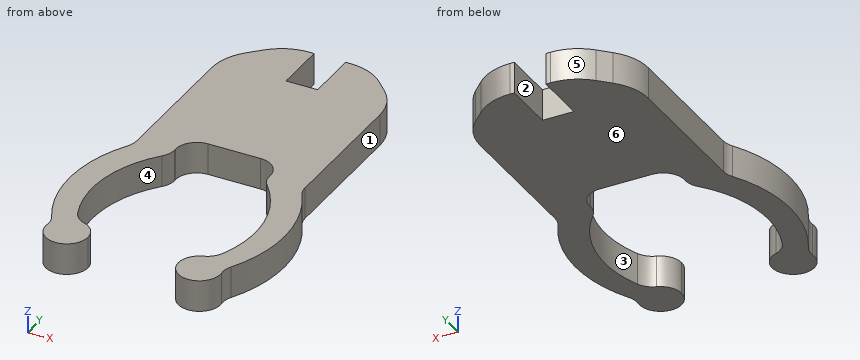
from build123d import *

# Parameters (mm, degrees)
F2_DEPTH = 1.5
F5_W     = 3
F5_H     = 5
F6_DEPTH = 25
F7_SIZE  = 4
F8_R     = 5
F9_R     = 2


with BuildPart() as f2:
    # F1 (on Top) → F2 (new body, symmetric)
    with BuildSketch(Plane.XY):
        with BuildLine():
            ThreePointArc((25.939839122, -44.6497348995), (25.3779596461, -43.9442064652), (24.8663520645, -43.2014167241))
            ThreePointArc((24.8663520645, -43.2014167241), (26.2921371989, -45.9579703612), (28.7, -44))
            ThreePointArc((28.7, -44), (28.0793670217, -42.5517781181), (26.6026533807, -42.0023704959))
            ThreePointArc((26.6026533807, -42.0023704959), (27.0242100762, -42.7170517529), (27.4984385882, -43.3979237417))
            ThreePointArc((27.4984385882, -43.3979237417), (27.6482717407, -43.6825402295), (27.7, -44))
            ThreePointArc((27.7, -44), (27.0462940384, -44.9381260251), (25.939839122, -44.6497348995))
        make_face()
        with BuildLine():
            ThreePointArc((27.4984385882, -43.3979237417), (26.0738018768, -43.2203360272), (25.939839122, -44.6497348995))
            ThreePointArc((25.939839122, -44.6497348995), (27.0462940384, -44.9381260251), (27.7, -44))
            ThreePointArc((27.7, -44), (27.6482717407, -43.6825402295), (27.4984385882, -43.3979237417))
        make_face()
        with BuildLine():
            ThreePointArc((26.6026533807, -42.0023704959), (25.5635084879, -42.3542822104), (24.8663520645, -43.2014167241))
            ThreePointArc((24.8663520645, -43.2014167241), (25.3779596461, -43.9442064652), (25.939839122, -44.6497348995))
            ThreePointArc((25.939839122, -44.6497348995), (26.0738018768, -43.2203360272), (27.4984385882, -43.3979237417))
            ThreePointArc((27.4984385882, -43.3979237417), (27.0242100762, -42.7170517529), (26.6026533807, -42.0023704959))
        make_face()
        with BuildLine():
            Line((28.5, -29), (25, -29))
            ThreePointArc((25, -29), (22.8225061684, -36.0808450853), (24.8663520645, -43.2014167241))
            ThreePointArc((24.8663520645, -43.2014167241), (25.5635084879, -42.3542822104), (26.6026533807, -42.0023704959))
            ThreePointArc((26.6026533807, -42.0023704959), (25.3965398825, -35.1867520093), (28.5, -29))
        make_face()
        Polygon((33, -9), (25, -9), (25, -29), (28.5, -29), (28.5, -26), (33, -26), align=None)
    extrude(amount=F2_DEPTH, both=True)


with BuildPart() as f2_1:
    # F3: moved
    add(f2.part.moved(Location((-33, 26, 0))))

    # F4: F2 across plane


with BuildPart() as f2_2:
    add(f2_1.part)
    add(f2_1.part.mirror(Plane.YZ))

    # F5 (on face) → F6 (cut)
    with BuildSketch(Plane.XY.offset(1.5)):
        with Locations((0, 14.5)):
            Rectangle(F5_W, F5_H)
    extrude(amount=-F6_DEPTH, mode=Mode.SUBTRACT)

    # F7
    f7_edges = [f2_2.edges().sort_by_distance(p)[0] for p in [
        (-8, 17, 0),
        (8, 17, 0),
    ]]
    chamfer(f7_edges, length=F7_SIZE)

    # F8
    f8_edges = [f2_2.edges().sort_by_distance(p)[0] for p in [
        (-8, 13, 0),
        (-4, 17, 0),
        (4, 17, 0),
        (8, 13, 0),
    ]]
    fillet(f8_edges, radius=F8_R)

    # F9
    f9_edges = [f2_2.edges().sort_by_distance(p)[0] for p in [
        (-8, -3, 0),
        (-4.5, -3, 0),
        (4.5, -3, 0),
        (8, -3, 0),
        (-4.5, 0, 0),
        (4.5, 0, 0),
        (-8.133648, -17.201417, 0),
        (-6.397347, -16.00237, 0),
        (8.133648, -17.201417, 0),
        (6.397347, -16.00237, 0),
    ]]
    fillet(f9_edges, radius=F9_R)


solid = f2_2.part
Geometry check sheet. Reference: the model listing, model coordinates, mm. Face numbers are marked on the shaded views. A direction names the side the tool comes from. Round coordinates to 2 decimals unless told otherwise and drop trailing zeros. Loops run counter-clockwise (first coordinate to the right, second up) from the corner with the lowest first, then second, coordinate; pieces in that order, holes last. Notation, with made-up numbers: (-13.5, 2.5) - (43.5, 2.5) arc R26 cw to (43.5, 25.5) - close; hole circle Ø4 at (-25.5, -28). An arc over 180 degrees is marked (long way). One line per question, with ' | ' between items. Start each with the question number.
1. Draft check along X on the marked faces 4, 5 and 6. Enter one of: released by +X, released by -X, zero draft, split by the parting line, or undercut.
2. Cross-section at A-A on x = 0.75. Record the cut outline in (y, z), then the cut area to 3 significant figures.
3. Scan lines: line 1 (X direction, y = 3.5, z = -0.1); line 2 (Y direction, x = 6.25, z = -1.05); line 3 (X direction, y = -7, z = -0.6). Record each from-to range of solid material in increasing order. Write a range as [from, to].
4. Cross-section at B-B on y = 5. Record the cut outline in (x, z).
5. Depth check by flat-ended pin: pin 1 (1.5 mm diameter, centred on y = 15, z = 0.5, fed in from +X); pin 2 (1.5 mm diameter, centred on y = 15.5, z = 0.5, fed in from -X). Enter the tip coordinate at first touch or a pass-through.
6. Tool access check on the marked faces 1, 2 and 3. Record the directions out of +Z, -Z, +X, -X, +Y, -Y that give a thin tool (end or side, any length) a straight path to the whole face; none if there is none.
Taken from the geometry:
1) face 4: undercut | face 5: released by -X | face 6: zero draft
2) outline: (0, -1.5) - (12, -1.5) - (12, 1.5) - (0, 1.5) - close | area: 36.0 mm²
3) line 1: [-8, 8] | line 2: [-20, -15.8], [-5.28, 14.75] | line 3: [-9.78, -7.05], [7.05, 9.78]
4) outline: (-8, -1.5) - (8, -1.5) - (8, 1.5) - (-8, 1.5) - close
5) pin 1: x = 6.74 | pin 2: x = -6.25
6) face 1: +Z, -Z, +X, +Y | face 2: +Z, -Z, +Y | face 3: +Z, -Z
